Verification items for the finished model (mm, model axes). Round coordinates to 2 decimals unless told otherwise and drop trailing zeros. Write each loop counter-clockwise with the first axis right and the second up, starting at its lowest first coordinate (ties: lowest second). Pieces come first, ordered by that corner, then holes.
from build123d import *

# Parameters (mm, degrees)
SKETCH_1_R           = 5
EXTRUDE_1_DEPTH      = 10
SKETCH_2_R           = 3
CUT_EXTRUDE_1_DEPTH  = 8
EXTRUDE_2_DEPTH      = 0.1
EXTRUDE_2_DEPTH_BACK = 10
SKETCH_4_W           = 8.393953891
SKETCH_4_H           = 2.961503145
SKETCH_5_W           = 8.393953891
SKETCH_5_H           = 10.1
EXTRUDE_3_DEPTH      = 30
EXTRUDE_4_DEPTH      = 0.1
EXTRUDE_4_DEPTH_BACK = 60
SKETCH_6_W           = 140
SKETCH_6_H           = 13.422298932


with BuildPart() as part:
    # 草图1 → 凸台-拉伸1 (new body)
    with BuildSketch(Plane.XY):
        Circle(SKETCH_1_R)
    extrude(amount=EXTRUDE_1_DEPTH)

    # 草图2 → 切除-拉伸1 (cut)
    with BuildSketch(Plane.XY.offset(10)):
        Circle(SKETCH_2_R)
    extrude(amount=-CUT_EXTRUDE_1_DEPTH, mode=Mode.SUBTRACT)

    # 草图4 → 凸台-拉伸2 (add, two sides: drawn at the far end of the back side and taken through both)
    with BuildSketch(Plane.XY.offset(10).offset(-EXTRUDE_2_DEPTH_BACK)):
        with Locations((0.020379312, 4.475569238)):
            Rectangle(SKETCH_4_W, SKETCH_4_H)
    extrude(amount=EXTRUDE_2_DEPTH + EXTRUDE_2_DEPTH_BACK)

    # 草图5 → 凸台-拉伸3 (add)
    with BuildSketch(Plane(origin=(0, 5.95632081, 0), x_dir=(1, 0, 0), z_dir=(0, 1, 0))):
        with Locations((0.020379312, -5.05)):
            Rectangle(SKETCH_5_W, SKETCH_5_H)
    extrude(amount=EXTRUDE_3_DEPTH)

    # 草图6 → 凸台-拉伸4 (add, two sides: drawn at the far end of the back side and taken through both)
    with BuildSketch(Plane.ZY.offset(4.176597634).offset(-EXTRUDE_4_DEPTH_BACK)):
        with Locations((-59.754924963, 31.401268081)):
            Rectangle(SKETCH_6_W, SKETCH_6_H)
    extrude(amount=EXTRUDE_4_DEPTH + EXTRUDE_4_DEPTH_BACK)


solid = part.part
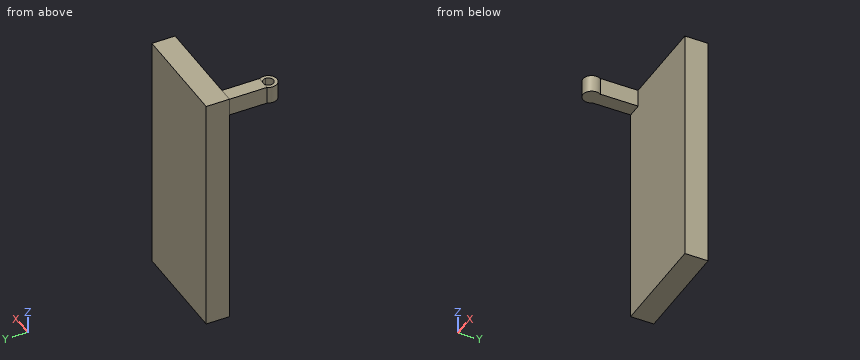
Q1. Depth check by flat-ended pin: P1, Ø4, axis at y = 30.5, z = -70, coming from the -X side; P2, Ø11, axis at x = 0.5, y = 11.5, coming from the -Z side; P3, Ø2.5, axis at x = -1.5, y = 16.5, coming from the +Z side. Enter the tip coordinate at first touch or a pass-through.
Recorded:
P1: stops at x = -4.28
P2: stops at z = 0
P3: stops at z = 10.1
Q2. Material ranges on line 1 along X through (y, z) = (0, 5); line 2 along X through (y, z) = (31, -54.5); line 3 along Z through (x, y) = (2, 1), recorded low to high.
Recorded:
line 1: x = -5 to -3, 3 to 5
line 2: x = -4.28 to 55.82
line 3: z = 0 to 2
Q3. Sectioned sample at A-A (z = -12). Enter the section's corners in (x, y).
Recorded:
outline: (-4.28, 24.69) - (55.82, 24.69) - (55.82, 38.11) - (-4.28, 38.11) - close
Q4. Sectioned sample at B-B (x = 26). Enter the section's corners in (y, z).
Recorded:
outline: (24.69, -129.75) - (38.11, -129.75) - (38.11, 10.25) - (24.69, 10.25) - close
